```python
from build123d import *

# Parameters (mm, degrees)
F0_W     = 50.8
F0_H     = 50.8
F1_DEPTH = 558.8


with BuildPart() as f1:
    # F0 (on Front) → F1 (new body)
    with BuildSketch(Plane.XZ):
        with Locations((0, -1.849517)):
            Rectangle(F0_W, F0_H)
        with BuildLine():
            Line((-22.098, 21.899483), (22.098, 21.899483))
            ThreePointArc((22.098, 21.899483), (23.265433, 21.415916), (23.749, 20.248483))
            Line((23.749, 20.248483), (23.749, -23.947517))
            ThreePointArc((23.749, -23.947517), (23.265433, -25.114951), (22.098, -25.598517))
            Line((22.098, -25.598517), (-22.098, -25.598517))
            ThreePointArc((-22.098, -25.598517), (-23.265433, -25.114951), (-23.749, -23.947517))
            Line((-23.749, -23.947517), (-23.749, 20.248483))
            ThreePointArc((-23.749, 20.248483), (-23.265433, 21.415916), (-22.098, 21.899483))
        make_face(mode=Mode.SUBTRACT)
    extrude(amount=F1_DEPTH)


solid = f1.part
```
Verification items for the finished model (mm, model axes). A direction names the side the tool comes from. Give positions to 0.01 mm unless a question says otherwise; leave off trailing zeros. Order: outer loops, then holes, each group sorted by start corner. A loop starts at its lowest first (then second) coordinate and runs counter-clockwise, first axis right, second up. Notation, with made-up numbers: M 22,56.5 L 60,56.5 A11 cw 60,70.5 Z; hole C 48,28.25 d2. An arc over 180 degrees is marked long. Answer in a Markdown table with one row per item. Add a question column.
Item 1: Scan lines: probe 1 along X at (y, z) = (-239, 3); probe 2 along Z at (x, y) = (-19, -100); probe 3 along X at (y, z) = (-278.5, 21). Record each from-to range of solid material in increasing order. Write a range as from..to.
Item 2: Section check B-B, the plane x = -13. Enter the section's corners in (y, z), and give its area (3 significant figures).
Item 3: Tool access check on faces 1 (the flat face through (0, -275, -25.599)), 2 (the flat face through (-2, -558.8, -26)). Record the directions out of +Z, -Z, +X, -X, +Y, -Y that give a thin tool (end or side, any length) a straight path to the whole face; none if there is none.
Item 4: Section check C-C, the plane y = -284.5. Enter the section's corners in (x, z), and give its area (3 significant figures).
Item 5: Mould release check, pull along Z, two halves, no side actions. Record for faces 3 (the flat face through (0, -275, 23.55)), 4 (the flat face through (23.749, -275, -2)), 5 (the flat face through (25.4, -275, -2)), 6 (the flat face through (0, -275, -27.25)): released by +Z, released by -Z, zero draft, split by the parting line, or undercut.
Item 6: Section check A-A, the plane z = 1. Enter the section's corners in (x, y), and give its area (3 significant figures).
Filled sheet:
| question | item | result |
|---|---|---|
| 1 | probe 1 | x = -25.4..-23.75, 23.75..25.4 |
| 1 | probe 2 | z = -27.25..-25.6, 21.9..23.55 |
| 1 | probe 3 | x = -25.4..-23.57, 23.57..25.4 |
| 2 | outline | M -558.8,-27.25 L 0,-27.25 L 0,-25.6 L -558.8,-25.6 Z; M -558.8,21.9 L 0,21.9 L 0,23.55 L -558.8,23.55 Z |
| 2 | area | 1,850 mm^2 |
| 3 | face 1 | +Y, -Y |
| 3 | face 2 | +Z, -Z, +X, -X, -Y |
| 4 | outline | M -25.4,-27.25 L 25.4,-27.25 L 25.4,23.55 L -25.4,23.55 Z; hole M -23.75,-23.95 A1.65 ccw -22.1,-25.6 L 22.1,-25.6 A1.65 ccw 23.75,-23.95 L 23.75,20.25 A1.65 ccw 22.1,21.9 L -22.1,21.9 A1.65 ccw -23.75,20.25 Z |
| 4 | area | 327 mm^2 |
| 5 | face 3 | released by +Z |
| 5 | face 4 | undercut |
| 5 | face 5 | zero draft |
| 5 | face 6 | released by -Z |
| 6 | outline | M -25.4,-558.8 L -23.75,-558.8 L -23.75,0 L -25.4,0 Z; M 23.75,-558.8 L 25.4,-558.8 L 25.4,0 L 23.75,0 Z |
| 6 | area | 1,850 mm^2 |
